from build123d import *

# Parameters (mm, degrees)
SKETCH3_W            = 60
SKETCH3_H            = 50
SKETCH3_R            = 4
SKETCH3_R_2          = 1.5
BOSS_EXTRUDE1_DEPTH  = 5
SKETCH4_R            = 2.5
CUT_EXTRUDE1_DEPTH   = 5
FILLET1_R            = 4
BOSS_EXTRUDE2_START  = 3
SKETCH5_R            = 6.5
SKETCH5_R_2          = 2.5
BOSS_EXTRUDE2_DEPTH  = 3
LPATTERN1_COUNT      = 2
LPATTERN1_PITCH      = 29
LPATTERN1_COUNT_DIR2 = 2
LPATTERN1_PITCH_DIR2 = 27


with BuildPart() as part:
    # Sketch3 → Boss-Extrude1 (new body)
    with BuildSketch(Plane(origin=(0, 0, 0), x_dir=(1, 0, 0), z_dir=(0, 1, 0))):
        with Locations((19.268140366, 2.797796233)):
            Rectangle(SKETCH3_W, SKETCH3_H)
        with Locations(Location((19.268140366, 2.797796233, 0), (0, 0, 270))):
            Circle(SKETCH3_R, mode=Mode.SUBTRACT)
        with Locations(Location((10.938140366, 2.797796233, 0), (0, 0, 270))):
            Circle(SKETCH3_R_2, mode=Mode.SUBTRACT)
        with Locations(Location((19.268140366, 11.127796233, 0), (0, 0, 270))):
            Circle(SKETCH3_R_2, mode=Mode.SUBTRACT)
        with Locations(Location((27.598140366, 2.797796233, 0), (0, 0, 270))):
            Circle(SKETCH3_R_2, mode=Mode.SUBTRACT)
        with Locations(Location((19.268140366, -5.532203767, 0), (0, 0, 270))):
            Circle(SKETCH3_R_2, mode=Mode.SUBTRACT)
    extrude(amount=BOSS_EXTRUDE1_DEPTH)

    # Sketch4 → Cut-Extrude1 (cut)
    with BuildSketch(Plane(origin=(0, 5, 0), x_dir=(1, 0, 0), z_dir=(0, 1, 0))):
        with Locations(Location((4.768140366, 16.297796233, 0), (0, 0, 270))):
            Circle(SKETCH4_R)
        with Locations(Location((33.768140366, 16.297796233, 0), (0, 0, 270))):
            Circle(SKETCH4_R)
        with Locations(Location((33.768140366, -10.702203767, 0), (0, 0, 270))):
            Circle(SKETCH4_R)
        with Locations(Location((4.768140366, -10.702203767, 0), (0, 0, 270))):
            Circle(SKETCH4_R)
    extrude(amount=-CUT_EXTRUDE1_DEPTH, mode=Mode.SUBTRACT)

    # Fillet1
    fillet1_edges = [part.edges().sort_by_distance(p)[0] for p in [
        (-10.731859634, 2.5, -27.797796233),
        (49.268140366, 2.5, -27.797796233),
        (49.268140366, 2.5, 22.202203767),
        (-10.731859634, 2.5, 22.202203767),
    ]]
    fillet(fillet1_edges, radius=FILLET1_R)

    # Sketch5 → Boss-Extrude2 (add)
    with BuildSketch(Plane(origin=(0, 5, 0), x_dir=(1, 0, 0), z_dir=(0, 1, 0)).offset(BOSS_EXTRUDE2_START)):
        with Locations(Location((33.768140366, 16.297796233, 0), (0, 0, 90))):
            Circle(SKETCH5_R)
        with Locations(Location((33.768140366, 16.297796233, 0), (0, 0, 270))):
            Circle(SKETCH5_R_2, mode=Mode.SUBTRACT)
    boss_extrude2 = extrude(amount=-BOSS_EXTRUDE2_DEPTH)

    # LPattern1: Boss-Extrude2 2 × 2
    with Locations(*[(-i * LPATTERN1_PITCH, 0, j * LPATTERN1_PITCH_DIR2) for i in range(LPATTERN1_COUNT) for j in range(LPATTERN1_COUNT_DIR2) if (i, j) != (0, 0)]):
        add(boss_extrude2)


solid = part.part
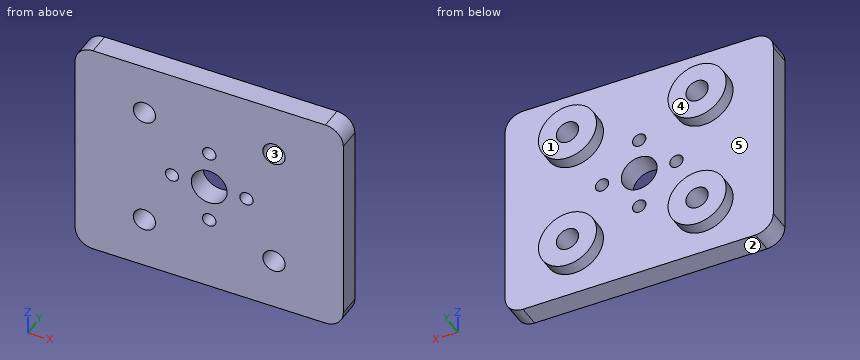
Design review of the part built by this model. Coordinates are the model's own, in mm. Face numbers are marked on the shaded views. A direction names the side the tool comes from. Coordinates: 2 decimals unless noted, no trailing zeros. Loops run counter-clockwise (first coordinate to the right, second up) from the corner with the lowest first, then second, coordinate; pieces in that order, holes last.
Item 1: Draft analysis for pull direction Z (two halves, no side actions). For the marked faces 1, 2 and 3, state which applies: pulls with the +Z half, pulls with the -Z half, needs draft (parallel to the pull), parting line crosses it, or undercut.
Completed:
face 1: needs draft
face 2: pulls with the -Z half
face 3: undercut
Item 2: Wall thickness on L1, parallel to X at y = 1, z = -17; L2, parallel to X at y = 6.5, z = 12.5; L3, parallel to X at y = 2, z = -15: over which ranges is each line inside the solid? List them lowest first.
Completed:
L1: x = -10.73 to 2.37, 7.17 to 31.37, 36.17 to 49.27
L2: x = -1.48 to 3.03, 6.51 to 11.01, 27.52 to 32.03, 35.51 to 40.01
L3: x = -10.73 to 2.63, 6.9 to 31.63, 35.9 to 49.27
Item 3: Add section B-B (z = -3.5). Write out the cut boundary in (x, y), and give its area (3 significant figures).
Completed:
outline: (-10.73, 0) - (9.61, 0) - (9.61, 5) - (-10.73, 5) - close; (12.26, 0) - (15.33, 0) - (15.33, 5) - (12.26, 5) - close; (23.21, 0) - (26.27, 0) - (26.27, 5) - (23.21, 5) - close; (28.92, 0) - (49.27, 0) - (49.27, 5) - (28.92, 5) - close
area: 234 mm2
Item 4: Clearance check with a flat-ended pin moving along its axis: pin 1 (6 mm diameter, centred on x = 15.5, z = -8.5, fed in from +Y). State where the tip first meets the part, or that it passes through.
Completed:
pin 1: stops at y = 5
Item 5: Add section A-A (x = 35). Write out the cut boundary in (y, z), and give its area (3 significant figures).
Completed:
outline: (0, -27.8) - (5, -27.8) - (5, -22.68) - (8, -22.68) - (8, -18.47) - (0, -18.47) - close; (0, -14.12) - (8, -14.12) - (8, -9.92) - (5, -9.92) - (5, 4.32) - (8, 4.32) - (8, 8.53) - (0, 8.53) - close; (0, 12.88) - (8, 12.88) - (8, 17.08) - (5, 17.08) - (5, 22.2) - (0, 22.2) - close
area: 257 mm2
Item 6: Add section C-C (y = 2.5). Give the number of separate pieces and of enclosed holes in the cut face, and give its area (3 significant figures).
Completed:
separate pieces: 1
enclosed holes: 9
area: 2,830 mm2
Item 7: Add section D-D (x = 22). Write out the cut boundary in (y, z), and give its area (3 significant figures).
Completed:
outline: (0, -27.8) - (5, -27.8) - (5, -5.72) - (0, -5.72) - close; (0, 0.12) - (5, 0.12) - (5, 22.2) - (0, 22.2) - close
area: 221 mm2
Item 8: For the marked faces 4 and 5, list the 3-axis set-ups (+Z, -Z, +X, -X, +Y, -Y) from which the entire face can be reached by the end or side of a thin tool; tool diameter is ignored.
Completed:
face 4: +Z, -Z, +X, -X, +Y
face 5: +Y
